For this review, take the finished solid that the model builds, in its own axes (mm). A direction names the side the tool comes from. Round coordinates to 2 decimals unless told otherwise and drop trailing zeros. Loops run counter-clockwise (first coordinate to the right, second up) from the corner with the lowest first, then second, coordinate; pieces in that order, holes last. Notation, with made-up numbers: (-14.75, -37.5) -> (25.25, -37.5) arc R27 cw to (25.25, -15.5) -> close; hole circle Ø10 at (39.25, 38). An arc over 180 degrees is marked (long way). Use one line per item in the form item = value. Start each with the question number.
from build123d import *

# Parameters (mm, degrees)
BOSS_EXTRUDE1_DEPTH = 15
FILLET1_R           = 7


with BuildPart() as part:
    # Sketch1 → Boss-Extrude1 (new body)
    with BuildSketch(Plane.XY):
        with BuildLine():
            Line((81.814228499, 422.253610621), (101.396155955, 422.253610621))
            ThreePointArc((101.396155955, 422.253610621), (112.002757673, 426.647008903), (116.396155955, 437.253610621))
            Line((116.396155955, 437.253610621), (116.396155955, 525.576232013))
            Line((116.396155955, 525.576232013), (128.396155955, 525.576232013))
            Line((128.396155955, 525.576232013), (128.396155955, 427.253610621))
            ThreePointArc((128.396155955, 427.253610621), (124.002757673, 416.647008903), (113.396155955, 412.253610621))
            Line((113.396155955, 412.253610621), (81.814228499, 412.253610621))
            Line((81.814228499, 412.253610621), (81.814228499, 422.253610621))
        make_face()
    extrude(amount=-BOSS_EXTRUDE1_DEPTH)

    # Fillet1
    fillet1_edges = [part.edges().sort_by_distance(p)[0] for p in [
        (122.396155955, 525.576232013, -15),
        (122.396155955, 525.576232013, 0),
    ]]
    fillet(fillet1_edges, radius=FILLET1_R)


solid = part.part
Item 1: Take a section at B-B on x = 124. Give the boundary of the cut face in (y, z).
Item 2: Wall thickness on line 1 (X direction, y = 484, z = -5.25); line 2 (Y direction, x = 94.5, z = -6); line 3 (X direction, y = 421.5, z = -2.5): over which ranges is each line inside the solid? List them lowest first.
Item 3: For P1, Ø4.5, axis at y = 463, z = -10.5, coming from the -X side; P2, Ø6, axis at x = 101, z = -11.5, coming from the +Y side; P3, Ø5, axis at x = 101, z = -5.5, coming from the +Y side, all flat-tipped, find the tip position at first contact; note any pin that passes through.
Item 4: Take a section at D-D on z = -5.75. Give the boundary of the cut face in (x, y).
Item 5: Machinability: for faces 1 (the flat face through (91, 422.254, -7)), 2 (the flat face through (81.814, 417, -7)), which of the approach directions +Z, -Z, +X, -X, +Y, -Y give a long, thin tool a straight path to every point of the face, cutting with its end or side? Answer none if there is none.
Item 6: Take a section at C-C on y = 473.5. Give the boundary of the cut face in (x, z), plus the area to 3 significant figures.
Item 7: Take a section at A-A on z = -1. Give the boundary of the cut face in (x, y).
Results:
q1.outline = (416.64, -15) -> (518.58, -15) arc R7 ccw to (525.58, -8) -> (525.58, -7) arc R7 ccw to (518.58, 0) -> (416.64, 0) -> close
q2.line_1 = 116.4 to 128.4
q2.line_2 = 412.25 to 422.25
q2.line_3 = 81.81 to 127.25
q3.P1 = 116.4
q3.P2 = 422.48
q3.P3 = 422.4
q4.outline = (81.81, 412.25) -> (113.4, 412.25) arc R15 ccw to (128.4, 427.25) -> (128.4, 525.46) -> (116.4, 525.46) -> (116.4, 437.25) arc R15 cw to (101.4, 422.25) -> (81.81, 422.25) -> close
q5.face_1 = +Z, -Z, -X, +Y
q5.face_2 = +Z, -Z, -X, +Y, -Y
q6.outline = (116.4, -15) -> (128.4, -15) -> (128.4, 0) -> (116.4, 0) -> close
q6.area = 180 mm2
q7.outline = (81.81, 412.25) -> (113.4, 412.25) arc R15 ccw to (128.4, 427.25) -> (128.4, 522.18) -> (116.4, 522.18) -> (116.4, 437.25) arc R15 cw to (101.4, 422.25) -> (81.81, 422.25) -> close
